Verification items for the finished model (mm, model axes). A direction names the side the tool comes from. Give positions to 0.01 mm unless a question says otherwise; leave off trailing zeros. Loops run counter-clockwise (first coordinate to the right, second up) from the corner with the lowest first, then second, coordinate; pieces in that order, holes last. Notation, with made-up numbers: (30.5, 75) -> (36.5, 75) arc R15 cw to (36.5, 103) -> close; hole circle Ø10 at (22, 83). An arc over 180 degrees is marked (long way). Answer in a Markdown table with one row per item. Add a question column.
Q1. Section check B-B on x = 2.5. Enter the section's corners in (y, z).
Q2. Set-up check for faces 1 (the face through (0, 22, 3)), 2 (the face through (0, 30, 3)), 3 (the face through (22.8, 12, 2)): record each of +Z, -Z, +X, -X, +Y, -Y from which the full face is reachable in a straight line by a thin tool's end or side.
Q3. Gauge pin test, flat ends, axial feed: P1, Ø1.3, axis at x = -19.5, y = 14.5, coming from the -Z side; P2, Ø3, axis at x = 26, y = 26, coming from the -Z side; P3, Ø2, axis at x = -26.5, y = 26.5, coming from the -Z side; P4, Ø2, axis at x = 21.5, y = 12, coming from the -Z side. Record the tip position at first contact, or that the pin passes through.
Q4. Release check for a two-part mould opening along Y. For faces 4 (the face through (-28.884, 28.843, 0.135)), 5 (the face through (0, 0, 0)), 6 (the face through (-17.2, 12, 2)) record: pulls with the +Y half, pulls with the -Y half, needs draft (parallel to the pull), parting line crosses it, or undercut.
Q5. Section check D-D on y = 12. Enter the section's corners in (x, z).
Q6. Section check A-A on y = -12. Enter the section's corners in (x, z), and give its area (3 significant figures).
Q7. Section check C-C on z = 1.5. Give the number of separate pieces and of enclosed holes in the cut face, and give its area (3 significant figures).
Q8. Material ranges on probe 1 along Y at (x, z) = (-26, 4.75); probe 2 along X at (y, z) = (12, 4.95); probe 3 along Y at (x, z) = (-10, 3.25), recorded low to high.
```python
from build123d import *

# Parameters (mm, degrees)
BOSS_EXTRUDE1_DEPTH = 6
SKETCH2_R           = 1.6
SKETCH2_R_2         = 6.5
SKETCH2_W           = 28
SKETCH2_H           = 20
CUT_EXTRUDE1_DEPTH  = 43.848570571
CUT_EXTRUDE2_START  = -1
SKETCH3_W           = 22.5
SKETCH3_H           = 16.5
CUT_EXTRUDE2_DEPTH  = 42.848570571
SKETCH4_W           = 14.5
SKETCH4_H           = 15.5
CUT_EXTRUDE3_DEPTH  = 43.720018727
CUT_EXTRUDE4_DEPTH  = 3
SKETCH6_W           = 5.6
SKETCH6_H           = 3.2
CUT_EXTRUDE5_DEPTH  = 0.4
SKETCH7_R           = 1.3
CUT_EXTRUDE6_DEPTH  = 5
CHAMFER2_SIZE       = 0.5


with BuildPart() as part:
    # Sketch1 → Boss-Extrude1 (new body)
    with BuildSketch(Plane.XY):
        with BuildLine():
            Line((-27, 30), (27, 30))
            ThreePointArc((27, 30), (29.121320344, 29.121320344), (30, 27))
            Line((30, 27), (30, -27))
            ThreePointArc((30, -27), (29.121320344, -29.121320344), (27, -30))
            Line((27, -30), (-27, -30))
            ThreePointArc((-27, -30), (-29.121320344, -29.121320344), (-30, -27))
            Line((-30, -27), (-30, 27))
            ThreePointArc((-30, 27), (-29.121320344, 29.121320344), (-27, 30))
        make_face()
    extrude(amount=BOSS_EXTRUDE1_DEPTH)

    # Sketch2 → Cut-Extrude1 (cut, through all)
    with BuildSketch(Plane.XY.offset(6)):
        with Locations((-20, 12)):
            Circle(SKETCH2_R)
        with Locations((20, 12)):
            Circle(SKETCH2_R)
        with Locations((15, -12)):
            Circle(SKETCH2_R_2)
        with Locations((0, 12)):
            Rectangle(SKETCH2_W, SKETCH2_H)
    extrude(amount=-CUT_EXTRUDE1_DEPTH, mode=Mode.SUBTRACT)

    # Sketch3 → Cut-Extrude2 (cut, through all)
    with BuildSketch(Plane.XY.offset(6).offset(CUT_EXTRUDE2_START)):
        with Locations((-11, -12)):
            Rectangle(SKETCH3_W, SKETCH3_H)
    extrude(amount=-CUT_EXTRUDE2_DEPTH, mode=Mode.SUBTRACT)

    # Sketch4 → Cut-Extrude3 (cut, through all)
    with BuildSketch(Plane(origin=(0, 0, 5), x_dir=(-1, 0, 0), z_dir=(0, 0, -1))):
        with Locations((14.5, -12)):
            Rectangle(SKETCH4_W, SKETCH4_H)
    extrude(amount=-CUT_EXTRUDE3_DEPTH, mode=Mode.SUBTRACT)

    # Sketch5 → Cut-Extrude4 (cut)
    with BuildSketch(Plane.XY):
        Polygon((-20, 8.766838493), (-17.2, 10.383419246), (-17.2, 13.616580754), (-20, 15.233161507), (-22.8, 13.616580754), (-22.8, 10.383419246), align=None)
        Polygon((20, 8.766838493), (22.8, 10.383419246), (22.8, 13.616580754), (20, 15.233161507), (17.2, 13.616580754), (17.2, 10.383419246), align=None)
    extrude(amount=CUT_EXTRUDE4_DEPTH, mode=Mode.SUBTRACT)

    # Sketch6 → Cut-Extrude5 (cut)
    with BuildSketch(Plane(origin=(0, 0, 3), x_dir=(-1, 0, 0), z_dir=(0, 0, -1))):
        with Locations((20, 12)):
            Rectangle(SKETCH6_W, SKETCH6_H)
        with Locations((-20, 12)):
            Rectangle(SKETCH6_W, SKETCH6_H)
    extrude(amount=-CUT_EXTRUDE5_DEPTH, mode=Mode.SUBTRACT)

    # Sketch7 → Cut-Extrude6 (cut)
    with BuildSketch(Plane(origin=(0, 0, 0), x_dir=(-1, 0, 0), z_dir=(0, 0, -1))):
        with Locations((-26, 26)):
            Circle(SKETCH7_R)
        with Locations((26, 26)):
            Circle(SKETCH7_R)
        with Locations((26, -26)):
            Circle(SKETCH7_R)
        with Locations((-26, -26)):
            Circle(SKETCH7_R)
    extrude(amount=-CUT_EXTRUDE6_DEPTH, mode=Mode.SUBTRACT)

    # Chamfer2
    chamfer2_edges = [part.edges().sort_by_distance(p)[0] for p in [
        (-29.121320344, 29.121320344, 6),
        (0, 30, 0),
        (29.121320344, 29.121320344, 0),
        (-30, 0, 6),
        (-29.121320344, -29.121320344, 6),
        (27.3, 26, 0),
        (-24.7, 26, 0),
        (-24.7, -26, 0),
        (27.3, -26, 0),
        (0, -30, 6),
        (29.121320344, -29.121320344, 6),
        (30, 0, 6),
        (29.121320344, 29.121320344, 6),
        (8.5, -12, 0),
        (8.5, -12, 6),
        (0, 30, 6),
        (30, 0, 0),
        (29.121320344, -29.121320344, 0),
        (0, -30, 0),
        (-29.121320344, -29.121320344, 0),
        (-30, 0, 0),
        (-29.121320344, 29.121320344, 0),
    ]]
    chamfer(chamfer2_edges, length=CHAMFER2_SIZE)


solid = part.part
```
Taken from the geometry:
| question | item | result |
|---|---|---|
| 1 | outline | (-30, 0.5) -> (-29.5, 0) -> (2, 0) -> (2, 6) -> (-29.5, 6) -> (-30, 5.5) -> close; (22, 0) -> (29.5, 0) -> (30, 0.5) -> (30, 5.5) -> (29.5, 6) -> (22, 6) -> close |
| 2 | face 1 | +Z, -Z |
| 2 | face 2 | +Z, -Z, +X, -X, +Y |
| 2 | face 3 | -Z |
| 3 | P1 | stops at z = 0 |
| 3 | P2 | stops at z = 0.3 |
| 3 | P3 | stops at z = 0.09 |
| 3 | P4 | stops at z = 3.4 |
| 4 | face 4 | pulls with the +Y half |
| 4 | face 5 | needs draft |
| 4 | face 6 | undercut |
| 5 | outline | (-30, 0.5) -> (-29.5, 0) -> (-22.8, 0) -> (-22.8, 3.4) -> (-21.6, 3.4) -> (-21.6, 6) -> (-29.5, 6) -> (-30, 5.5) -> close; (-18.4, 3.4) -> (-17.2, 3.4) -> (-17.2, 0) -> (-14, 0) -> (-14, 6) -> (-18.4, 6) -> close; (14, 0) -> (17.2, 0) -> (17.2, 3.4) -> (18.4, 3.4) -> (18.4, 6) -> (14, 6) -> close; (21.6, 3.4) -> (22.8, 3.4) -> (22.8, 0) -> (29.5, 0) -> (30, 0.5) -> (30, 5.5) -> (29.5, 6) -> (21.6, 6) -> close |
| 6 | outline | (-30, 0.5) -> (-29.5, 0) -> (-22.25, 0) -> (-22.25, 5) -> (-21.75, 5) -> (-21.75, 6) -> (-29.5, 6) -> (-30, 5.5) -> close; (-7.25, 5) -> (0.25, 5) -> (0.25, 0) -> (8, 0) -> (8.5, 0.5) -> (8.5, 5.5) -> (8, 6) -> (-7.25, 6) -> close; (21.5, 0.5) -> (22, 0) -> (29.5, 0) -> (30, 0.5) -> (30, 5.5) -> (29.5, 6) -> (22, 6) -> (21.5, 5.5) -> close |
| 6 | area | 154 mm² |
| 7 | separate pieces | 1 |
| 7 | enclosed holes | 9 |
| 7 | area | 2,450 mm² |
| 8 | probe 1 | y = -30 to -27.3, -24.7 to 24.7, 27.3 to 30 |
| 8 | probe 2 | x = -30 to -21.6, -18.4 to -14, 14 to 18.4, 21.6 to 30 |
| 8 | probe 3 | y = -30 to -20.25, -3.75 to 2, 22 to 30 |
